```python
from build123d import *

# Parameters (mm, degrees)
F0_W      = 88.8
F0_H      = 26
F1_DEPTH  = 60
F3_DEPTH  = 45
F4_R      = 2
F5_W      = 88.9
F5_H      = 40
F6_DEPTH  = 10
F8_DEPTH  = 10
F9_R      = 2
F10_W     = 89
F10_H     = 45
F11_DEPTH = 15
F13_DEPTH = 5
F14_R     = 2
F15_R     = 4.6723110677
F15_R_2   = 4
F16_DEPTH = 85.001
F17_W     = 79.5239582658
F17_H     = 118.802215904
F18_DEPTH = 80
F19_R     = 3
F20_DEPTH = 3
F20_TAPER = -3
F21_DEPTH = 3
F21_TAPER = 3
F22_R     = 5.0890490665
F23_DEPTH = 25
F23_TAPER = -3


with BuildPart() as f1:
    # F0 (on Top) → F1 (new body)
    with BuildSketch(Plane.XY):
        Rectangle(F0_W, F0_H)
    extrude(amount=F1_DEPTH)

    # F2 (on face) → F3 (cut)
    with BuildSketch(Plane(origin=(0, 0, 0), x_dir=(1, 0, 0), z_dir=(0, 0, -1))):
        Polygon((-17.5, -7.6945363638), (0, -8), (17.5, -7.6945363638), (17.5, 7.6945363638), (0, 8), (-17.5, 7.6945363638), align=None)
    extrude(amount=-F3_DEPTH, mode=Mode.SUBTRACT)

    # F4
    f4_edges = [f1.edges().sort_by_distance(p)[0] for p in [
        (-17.5, 7.694536, 22.5),
        (-17.5, -7.694536, 22.5),
        (17.5, -7.694536, 22.5),
        (17.5, 7.694536, 22.5),
    ]]
    fillet(f4_edges, radius=F4_R)

    # F5 (on face) → F6 (join)
    with BuildSketch(Plane(origin=(0, 0, 0), x_dir=(1, 0, 0), z_dir=(0, 0, -1))):
        Rectangle(F5_W, F5_H)
    extrude(amount=F6_DEPTH)

    # F7 (on face) → F8 (cut)
    with BuildSketch(Plane(origin=(0, 0, -10), x_dir=(1, 0, 0), z_dir=(0, 0, -1))):
        Polygon((-20, -10.1508987014), (0, -10.5), (20, -10.1508987014), (20, 10.1508987014), (0, 10.5), (-20, 10.1508987014), align=None)
    extrude(amount=-F8_DEPTH, mode=Mode.SUBTRACT)

    # F9
    f9_edges = [f1.edges().sort_by_distance(p)[0] for p in [
        (-20, 10.150899, -5),
        (-20, -10.150899, -5),
        (20, 10.150899, -5),
        (20, -10.150899, -5),
    ]]
    fillet(f9_edges, radius=F9_R)

    # F10 (on face) → F11 (join)
    with BuildSketch(Plane(origin=(0, 0, -10), x_dir=(1, 0, 0), z_dir=(0, 0, -1))):
        Rectangle(F10_W, F10_H)
    extrude(amount=F11_DEPTH)

    # F12 (on face) → F13 (cut)
    with BuildSketch(Plane.XY.offset(-10)):
        Polygon((-39.5, -16.5605249353), (0, -17.25), (39.5, -16.5605249353), (39.5, 16.5605249353), (0, 17.25), (-39.5, 16.5605249353), align=None)
    extrude(amount=-F13_DEPTH, mode=Mode.SUBTRACT)

    # F14
    f14_edges = [f1.edges().sort_by_distance(p)[0] for p in [
        (-39.5, 16.560525, -12.5),
        (-39.5, -16.560525, -12.5),
        (39.5, -16.560525, -12.5),
        (39.5, 16.560525, -12.5),
    ]]
    fillet(f14_edges, radius=F14_R)

    # F15 (on face) → F16 (cut, through all)
    with BuildSketch(Plane.XY.offset(60)):
        with Locations((-27.5, 0)):
            Circle(F15_R)
        with Locations((27.5, 0)):
            Circle(F15_R_2)
    extrude(amount=-F16_DEPTH, mode=Mode.SUBTRACT)

    # F17 (on Right) → F18 (cut)
    with BuildSketch(Plane.YZ):
        with Locations((3.9665214717, 9.8679382354)):
            Rectangle(F17_W, F17_H)
    extrude(amount=-F18_DEPTH, mode=Mode.SUBTRACT)

    # F19 (on face) → F20 (join)
    with BuildSketch(Plane(origin=(0, 0, 0), x_dir=(0, -1, 0), z_dir=(-1, 0, 0))):
        with Locations((8.2831978798, 53.2280467451)):
            Circle(F19_R)
        with Locations((0, -20.896807313)):
            Circle(F19_R)
        with Locations((-8.2831978798, 53.2280467451)):
            Circle(F19_R)
    extrude(amount=-F20_DEPTH, taper=F20_TAPER)

    # F19 (on face) → F21 (cut)
    with BuildSketch(Plane(origin=(0, 0, 0), x_dir=(0, -1, 0), z_dir=(-1, 0, 0))):
        with Locations((8.2831978798, 53.2280467451)):
            Circle(F19_R)
        with Locations((0, -20.896807313)):
            Circle(F19_R)
        with Locations((-8.2831978798, 53.2280467451)):
            Circle(F19_R)
    extrude(amount=-F21_DEPTH, taper=F21_TAPER, mode=Mode.SUBTRACT)

    # F22 (on face) → F23 (cut)
    with BuildSketch(Plane(origin=(0, 0, 45), x_dir=(1, 0, 0), z_dir=(0, 0, -1))):
        Circle(F22_R)
    extrude(amount=-F23_DEPTH, taper=F23_TAPER, mode=Mode.SUBTRACT)


solid = f1.part
```
Source: CAD feature listing. Evaluate the final solid. Frame: model axes, mm. A direction names the side the tool comes from. Coordinates: 2 decimals unless noted, no trailing zeros. Loops run counter-clockwise (first coordinate to the right, second up) from the corner with the lowest first, then second, coordinate; pieces in that order, holes last. Notation, with made-up numbers: (80, -26) -> (125, -26) arc R9 cw to (125, -17) -> close; hole circle Ø5 at (-15, -37). An arc over 180 degrees is marked (long way). One line per item, written item: value. Start each with the question number.
Q1. Section query C-C, the plane y = 0. Return the cut outline in (x, z), and give its area (3 significant figures).
Q2. Section query A-A, the plane x = 27.5. Return the cut outline in (y, z), and give its area (3 significant figures).
Q3. Section query B-B, the plane z = 23. Return the cut outline in (x, y).
Q4. Line query: line 1 along Z through (x, y) = (33, 14.5); line 2 along Z through (x, y) = (14, 3); line 3 along Y through (x, z) = (27.5, -19.75). Output: solid intervals per line, ascending.
Q5. Contact query for flat-ended pins moving along their axis: P1, Ø3, axis at x = 15.5, y = -17.5, coming from the +Z side; P2, Ø5, axis at x = 37.5, z = 20, coming from the +Y side; P3, Ø3.5, axis at y = 1, z = 30.5, coming from the -X side; P4, Ø4.5, axis at y = -1, z = -20, coming from the -X side. Output: stop coordinate, or through.
Q6. Mould query, pull axis Z, two halves, no side actions, for faces 1 (the face through (17.5, 0, 22)), 2 (the face through (1.854, -11.052, 54.1)), 3 (the face through (44.4, 0, 30)), 4 (the face through (5.486, 0.121, 52.605)). Classes: pulls with the +Z half, pulls with the -Z half, needs draft (parallel to the pull), parting line crosses it, or undercut.
Q7. Set-up query: faces 5 (the face through (22, 13, 30)), 6 (the face through (18, 1, 0)), 7 (the face through (0, 8.2, 5.1)). Return all of +Z, -Z, +X, -X, +Y, -Y with unobstructed straight access to the full face (end or side cutting, diameter ignored); none if empty.
Results:
1. outline: (0, -25) -> (23.5, -25) -> (23.5, -15) -> (0, -15) -> (0, -17.9) -> (3, -18.05) -> (3, -23.74) -> (0, -23.9) -> close; (5.09, 45) -> (17.5, 45) -> (17.5, 0) -> (20, 0) -> (20, -10) -> (23.5, -10) -> (23.5, 60) -> (5.88, 60) -> close; (31.5, -25) -> (44.5, -25) -> (44.5, -10) -> (44.45, -10) -> (44.45, 0) -> (44.4, 0) -> (44.4, 60) -> (31.5, 60) -> (31.5, -10) -> (39.5, -10) -> (39.5, -15) -> (31.5, -15) -> close
1. area: 1,850 mm^2
2. outline: (-22.5, -25) -> (-4, -25) -> (-4, -15) -> (-16.77, -15) -> (-16.77, -10) -> (-4, -10) -> (-4, 60) -> (-13, 60) -> (-13, 0) -> (-20, 0) -> (-20, -10) -> (-22.5, -10) -> close; (4, -25) -> (22.5, -25) -> (22.5, -10) -> (20, -10) -> (20, 0) -> (13, 0) -> (13, 60) -> (4, 60) -> (4, -10) -> (16.77, -10) -> (16.77, -15) -> (4, -15) -> close
2. area: 1,830 mm^2
3. outline: (0, -13) -> (44.4, -13) -> (44.4, 13) -> (0, 13) -> (0, 8) -> (15.53, 7.73) arc R2 cw to (17.5, 5.73) -> (17.5, -5.73) arc R2 cw to (15.53, -7.73) -> (0, -8) -> close; hole circle Ø8 at (27.5, 0)
4. line 1: -25 to -15, -10 to 0
4. line 2: -25 to -15, 45 to 60
4. line 3: -22.5 to -4, 4 to 22.5
5. P1: z = 0
5. P2: y = 13
5. P3: x = 17.5
5. P4: x = 0
6. face 1: undercut
6. face 2: undercut
6. face 3: needs draft
6. face 4: pulls with the +Z half
7. face 5: +Z, +X, -X, +Y
7. face 6: -X
7. face 7: +Z, -Z, -X, +Y, -Y
